For this review, take the finished solid that the model builds, in its own axes (mm). A direction names the side the tool comes from. Coordinates: 2 decimals unless noted, no trailing zeros. Write each loop counter-clockwise with the first axis right and the second up, starting at its lowest first coordinate (ties: lowest second). Pieces come first, ordered by that corner, then holes. Notation, with made-up numbers: (-17, 3.5) -> (12, 3.5) arc R22 ccw to (12, 38.5) -> close; hole circle Ø2 at (-2.75, 14.5). An arc over 180 degrees is marked (long way). One line per item, written item: value. Start each with the question number.
1) Add section D-D (z = -15.5). State the section outline as (x, y) points.
2) For probe 1 along Z at (x, y) = (0, -10.25); probe 2 along X at (y, z) = (-17, 0); probe 3 along Y at (x, z) = (4.5, 7.5), list the stretches that pass through material, from the lowest coordinate up. Write a range as from..to.
3) For pin 1 Ø6 at (x, y) = (-5.5, -6) entering from -Z; pin 2 Ø2 at (x, y) = (-5.5, -5.5) entering from +Z; pin 3 Ø2 at (x, y) = (-2, -3) entering from -Z, all flat-tipped, find the tip position at first contact; note any pin that passes through.
4) Mouldability with a two-part tool opening along X and no side actions: class faces 4 (the cylindrical face through (3.1, -12.6, -0.1)), 5 (the flat face through (8.01, -6.82, -14.14)), 6 (the flat face through (-8.239, -6.818, -14.007)) as released by +X, released by -X, zero draft, split by the parting line, or undercut.
5) Add section C-C (y = 4). State the section outline as (x, z) points, and give its area (3 significant figures).
6) Add section B-B (z = 0). State the section outline as (x, y) points.
7) Add section A-A (y = -15.5). State the section outline as (x, z) points.
8) Machinability: for faces 1 (the flat face through (0, -2, 0)), 2 (the flat face through (8.239, -6.818, 14.007)), 3 (the flat face through (-2.618, -13, 0)), which of the approach directions +Z, -Z, +X, -X, +Y, -Y give a long, thin tool a straight path to every point of the face, cutting with its end or side? Answer none if there is none.
from build123d import *

# Parameters (mm, degrees)
SKETCH1_R           = 11.35
BOSS_EXTRUDE1_DEPTH = 6
BOSS_EXTRUDE4_DEPTH = 20
CUT_EXTRUDE2_DEPTH  = 15
CHAMFER3_SIZE       = 2
CHAMFER3_SIZE2      = 3.464101615
CUT_EXTRUDE4_START  = -2
SKETCH9_R           = 11.35
CUT_EXTRUDE4_DEPTH  = 2


with BuildPart() as part:
    # Sketch1 → Boss-Extrude1 (new body)
    with BuildSketch(Plane(origin=(0, 0, 0), x_dir=(1, 0, 0), z_dir=(0, 1, 0))):
        Polygon((16.25, 9.381941874), (0, 18.763883749), (-16.25, 9.381941874), (-16.25, -9.381941874), (0, -18.763883749), (16.25, -9.381941874), align=None)
        with Locations(Location((0, 0, 0), (0, 0, 270))):
            Circle(SKETCH1_R, mode=Mode.SUBTRACT)
    extrude(amount=BOSS_EXTRUDE1_DEPTH)

    # Sketch5 → Boss-Extrude4 (add)
    with BuildSketch(Plane.XZ):
        Polygon((16.25, 9.381941874), (0, 18.763883749), (-16.25, 9.381941874), (-16.25, -9.381941874), (0, -18.763883749), (16.25, -9.381941874), align=None)
    extrude(amount=BOSS_EXTRUDE4_DEPTH)

    # Sketch6 → Cut-Extrude2 (cut)
    with BuildSketch(Plane.XZ.offset(20)):
        with BuildLine():
            Line((-2.618090908, 1.66), (-2.618090908, -1.66))
            ThreePointArc((-2.618090908, -1.66), (3.1, 0), (-2.618090908, 1.66))
        make_face()
    extrude(amount=-CUT_EXTRUDE2_DEPTH, mode=Mode.SUBTRACT)

    # Chamfer3
    chamfer3_edges = [part.edges().sort_by_distance(p)[0] for p in [
        (0, 6, -11.35),
    ]]
    chamfer3_side = [part.faces().sort_by_distance(p)[0] for p in [
        (7.87677715, 6, -13.642978223),
    ]]
    chamfer(chamfer3_edges, length=CHAMFER3_SIZE, length2=CHAMFER3_SIZE2, reference=chamfer3_side[0])

    # Sketch9 → Cut-Extrude4 (cut)
    with BuildSketch(Plane(origin=(0, 0, 0), x_dir=(1, 0, 0), z_dir=(0, 1, 0)).offset(CUT_EXTRUDE4_START)):
        with Locations(Location((0, 0, 0), (0, 0, 270))):
            Circle(SKETCH9_R)
    extrude(amount=CUT_EXTRUDE4_DEPTH, mode=Mode.SUBTRACT)


solid = part.part
Numbers:
1. outline: (-5.65, -20) -> (5.65, -20) -> (5.65, 6) -> (-5.65, 6) -> close
2. probe 1: -18.76..-3.1, 3.1..18.76
2. probe 2: -16.25..-2.62, 3.1..16.25
2. probe 3: -20..-2
3. pin 1: z = -17.32
3. pin 2: z = 16.17
3. pin 3: z = -18.19
4. face 4: undercut
4. face 5: released by +X
4. face 6: released by -X
5. outline: (-16.25, -9.38) -> (0, -18.76) -> (16.25, -9.38) -> (16.25, 9.38) -> (0, 18.76) -> (-16.25, 9.38) -> close; hole circle Ø24.39 at (0, 0)
5. area: 448 mm²
6. outline: (-16.25, -20) -> (-2.62, -20) -> (-2.62, -5) -> (3.1, -5) -> (3.1, -20) -> (16.25, -20) -> (16.25, 6) -> (13.35, 6) -> (11.35, 2.54) -> (11.35, -2) -> (-11.35, -2) -> (-11.35, 2.54) -> (-13.35, 6) -> (-16.25, 6) -> close
7. outline: (-16.25, -9.38) -> (0, -18.76) -> (16.25, -9.38) -> (16.25, 9.38) -> (0, 18.76) -> (-16.25, 9.38) -> close; hole (-2.62, -1.66) arc R3.1 ccw (long way) to (-2.62, 1.66) -> close
8. face 1: +Y
8. face 2: +Z, +X, +Y, -Y
8. face 3: -Y
